The listing builds one solid part. Answer for the finished solid, in the listing's coordinates (mm). A direction names the side the tool comes from. Coordinates: 2 decimals unless noted, no trailing zeros. Order: outer loops, then holes, each group sorted by start corner. A loop starts at its lowest first (then second) coordinate and runs counter-clockwise, first axis right, second up. Notation, with made-up numbers: (-8.75, 51.5) - (11.25, 51.5) arc R19 ccw to (11.25, 81.5) - close; hole circle Ø8 at (77, -26). An arc over 180 degrees is marked (long way). Use one line per item in the form item = value. Start each with the question number.
Item 1: Consider line 1 along Z through (x, y) = (-73.5, -11); line 2 along Z through (x, y) = (-61.5, 7.5); line 3 along X through (y, z) = (-12, 88). Determine where each line is inside the solid, lowest interval first. Write a range as [from, to].
Item 2: Section D-D, the plane x = 110.5 is taken. Write down the section's boundary in (y, z).
Item 3: The mould has two halves that part along X. Classify faces 1 (the flat face through (30.043, -23.751, 87.881)), 2 (the flat face through (0, -29.759, 67)), 3 (the cylindrical face through (-127.27, 3.93, 19.11)): released by +X, released by -X, zero draft, split by the parting line, or undercut.
Item 4: A tool of negligible diameter and unlimited length cuts with its end or side. For faces 4 (the flat face through (-121, 2.366, 14)), 5 (the flat face through (-114.166, 3.931, 20.891)), 6 (the flat face through (-13.976, -24.135, 72.232)), 7 (the flat face through (15.756, -24.135, 85.592)), 8 (the flat face through (-121, 5.541, 14)), from which of +Z, -Z, +X, -X, +Y, -Y can it reach the whole face along a straight path? Write none if from no direction.
Item 5: Section C-C, the plane y = -12 is taken. Write down the section's boundary in (x, z).
Item 6: Each of these flat-tipped pins is pushed along its axis until it touches: pin 1 Ø1 at (x, y) = (49.5, -13) entering from +Z; pin 2 Ø4 at (x, y) = (69, -19.5) entering from -Z; pin 3 Ø10 at (y, z) = (-25, 41.5) entering from +X. Where does it stop, or does it pass through?
Item 7: Section B-B, the plane z = 0.5 is taken. Write down the section's boundary in (x, y).
Item 8: Section A-A, the plane y = 20 is taken. Write down the section's boundary in (x, z), and give its area (3 significant figures).
from build123d import *

# Parameters (mm, degrees)
BOSS_EXTRUDE1_DEPTH      = 25.4
BOSS_EXTRUDE1_DEPTH_BACK = 38.1
SKETCH8_W                = 123.535434654
SKETCH8_H                = 17.820393788
SKETCH8_W_2              = 107.648650008
SKETCH8_H_2              = 18.69081023
SKETCH8_W_3              = 70.279057637
SKETCH8_H_3              = 8.745584685
CUT_EXTRUDE8_DEPTH       = 249.85459317
SKETCH9_W                = 13.97
SKETCH9_H                = 3.175
BOSS_EXTRUDE2_DEPTH      = 19.05
SKETCH10_R               = 3.5
SKETCH10_R_2             = 3.33435983
CUT_EXTRUDE9_DEPTH       = 193.549453602
SKETCH11_R               = 3.3
BOSS_EXTRUDE3_DEPTH      = 3.175


with BuildPart() as part:
    # Sketch1 → Boss-Extrude1 (new, two sides: drawn at the far end of the back side and taken through both)
    with BuildSketch(Plane(origin=(0, 0, 0), x_dir=(1, 0, 0), z_dir=(0, 1, 0)).offset(-BOSS_EXTRUDE1_DEPTH_BACK)):
        with BuildLine():
            Line((75.173258544, -98.513613558), (-56.782466528, -39.220463143))
            Line((-56.782466528, -39.220463143), (-69.080642984, -33.693819057))
            Line((-69.080642984, -33.693819057), (-80.694369412, -27.627832989))
            ThreePointArc((-80.694369412, -27.627832989), (-118.690304786, 60.820348405), (-41.597550485, 118.469972265))
            Line((-41.597550485, 118.469972265), (-40.510743974, 121.612378267))
            ThreePointArc((-40.510743974, 121.612378267), (-121.611751141, 62.177923058), (-82.302619901, -30.367309292))
            Line((-82.302619901, -30.367309292), (-70.352378469, -36.603743496))
            Line((-70.352378469, -36.603743496), (73.849161484, -101.399443673))
            ThreePointArc((73.849161484, -101.399443673), (128.866936987, -89.667676037), (132.52114904, -33.531798673))
            Line((132.52114904, -33.531798673), (129.87034504, -35.279329261))
            ThreePointArc((129.87034504, -35.279329261), (126.457174239, -87.60035304), (75.173258544, -98.513613558))
        make_face()
    extrude(amount=BOSS_EXTRUDE1_DEPTH + BOSS_EXTRUDE1_DEPTH_BACK)

    # Sketch8 → Cut-Extrude8 (cut, through all)
    with BuildSketch(Plane(origin=(-26.544057216, 0, 59.073270551), x_dir=(0.9121462285238172, 0, 0.4098649262742256), z_dir=(-0.4098649262742256, 0, 0.9121462285238172))):
        with Locations((-97.740996954, 18.372591372)):
            Rectangle(SKETCH8_W, SKETCH8_H)
        with Locations((117.247557269, -29.159427294)):
            Rectangle(SKETCH8_W_2, SKETCH8_H_2)
        with Locations((28.283703447, -34.132040067)):
            Rectangle(SKETCH8_W_3, SKETCH8_H_3)
    extrude(amount=-CUT_EXTRUDE8_DEPTH, mode=Mode.SUBTRACT)

    # Sketch9 → Boss-Extrude2 (add)
    with BuildSketch(Plane(origin=(-25.503000303, 0, 56.756419131), x_dir=(0.9121462285238173, 0, 0.40986492627422544), z_dir=(-0.40986492627422544, 0, 0.9121462285238173))):
        with Locations((56.438232265, -24.112299079)):
            Rectangle(SKETCH9_W, SKETCH9_H)
        with Locations((23.842597685, -24.112299079)):
            Rectangle(SKETCH9_W, SKETCH9_H)
    extrude(amount=BOSS_EXTRUDE2_DEPTH)

    # Sketch10 → Cut-Extrude9 (cut, through all)
    with BuildSketch(Plane(origin=(0, -25.699799079, 0), x_dir=(-1, 0, 0), z_dir=(0, -1, 0))):
        with Locations(Location((-21.260331788, -90.924752525, 0), (0, 0, 180))):
            Circle(SKETCH10_R)
        with Locations(Location((8.708938333, -77.458323235, 0), (0, 0, 180))):
            Circle(SKETCH10_R_2)
    extrude(amount=-CUT_EXTRUDE9_DEPTH, mode=Mode.SUBTRACT)

    # Sketch11 → Boss-Extrude3 (add)
    with BuildSketch(Plane(origin=(0, 2.365700518, 0), x_dir=(1, 0, 0), z_dir=(0, 1, 0))):
        with BuildLine():
            Line((-137.515282661, -12.448119592), (-117.841020701, 8.538369727))
            ThreePointArc((-117.841020701, 8.538369727), (-111.239130232, -3.699946448), (-102.640289142, -14.627950496))
            Line((-102.640289142, -14.627950496), (-126.018526364, -27.331725219))
            ThreePointArc((-126.018526364, -27.331725219), (-138.10436789, -24.785259853), (-137.515282661, -12.448119592))
        make_face()
        with Locations(Location((-130.566346327, -18.962558081, 0), (0, 0, 180))):
            Circle(SKETCH11_R, mode=Mode.SUBTRACT)
    extrude(amount=BOSS_EXTRUDE3_DEPTH)


solid = part.part
Response:
q1.line_1 = [-115.93, -112.5], [31.39, 34.96]
q1.line_2 = [-119.66, -116.4], [37.1, 40.58]
q1.line_3 = [44.03, 51.78], [126.11, 130.24]
q2.outline = (-19.81, 99.2) - (25.4, 99.2) - (25.4, 102.63) - (-19.81, 102.63) - close
q3.face_1 = released by +X
q3.face_2 = zero draft
q3.face_3 = undercut
q4.face_4 = +Z, -X, -Y
q4.face_5 = +Z, +Y, -Y
q4.face_6 = -X, +Y, -Y
q4.face_7 = +Y, -Y
q4.face_8 = +Z, -X, +Y
q5.outline = (-82.3, 30.37) arc R80.96 ccw to (-40.51, -121.61) - (-41.6, -118.47) arc R77.78 cw to (-80.69, 27.63) - (-69.08, 33.69) - (-56.78, 39.22) - (75.17, 98.51) arc R43.43 cw to (129.87, 35.28) - (132.52, 33.53) arc R46.61 ccw to (73.85, 101.4) - (-70.35, 36.6) - close
q6.pin_1 = 90.68
q6.pin_2 = 94.84
q6.pin_3 = -40.58
q7.outline = (-126.31, 2.37) - (-113.23, 2.37) - (-113.23, -38.1) - (-109.52, -38.1) - (-109.52, 9.46) - (-113.23, 9.46) - (-113.23, 5.54) - (-126.31, 5.54) - close
q8.outline = (-58.32, 42.01) - (-57.01, 39.12) - (-56.78, 39.22) - (75.17, 98.51) arc R43.43 cw to (129.87, 35.28) - (132.52, 33.53) arc R46.61 ccw to (73.85, 101.4) - close
q8.area = 831 mm2
